Work out the finished part from the listing and answer in its coordinate system (mm). A direction names the side the tool comes from. Round coordinates to 2 decimals unless told otherwise and drop trailing zeros. Write each loop counter-clockwise with the first axis right and the second up, starting at its lowest first coordinate (ties: lowest second). Pieces come first, ordered by that corner, then holes.
from build123d import *

# Parameters (mm, degrees)
SKETCH_263_W        = 2284
SKETCH_263_H        = 90
EXTRUDE_4_DEPTH     = 8
SKETCH_3_W          = 2284
SKETCH_3_H          = 9
EXTRUDE_5_DEPTH     = 72
SKETCH_4_R          = 11
CUT_EXTRUDE_2_DEPTH = 2287.835586569


with BuildPart() as part:
    # Sketch 263 → 拉伸4 (new body)
    with BuildSketch(Plane.XY):
        with Locations((1142, 45)):
            Rectangle(SKETCH_263_W, SKETCH_263_H)
    extrude(amount=EXTRUDE_4_DEPTH)

    # 草图3 → 拉伸5 (add)
    with BuildSketch(Plane.XY.offset(8)):
        with Locations((1142, 4.5)):
            Rectangle(SKETCH_3_W, SKETCH_3_H)
    extrude(amount=EXTRUDE_5_DEPTH)

    # 草图4 → 切除-拉伸2 (cut, through all)
    with BuildSketch(Plane(origin=(0, 9, 0), x_dir=(1, 0, 0), z_dir=(0, 1, 0))):
        with Locations(Location((39.95, -40, 0), (0, 0, 270))):
            Circle(SKETCH_4_R)
        with Locations(Location((109.95, -40, 0), (0, 0, 270))):
            Circle(SKETCH_4_R)
        with Locations(Location((2174.05, -40, 0), (0, 0, 270))):
            Circle(SKETCH_4_R)
        with Locations(Location((2244.05, -40, 0), (0, 0, 270))):
            Circle(SKETCH_4_R)
    extrude(amount=-CUT_EXTRUDE_2_DEPTH, mode=Mode.SUBTRACT)


solid = part.part
Q1. Find the intervals of material crossed by L1, parallel to X at y = 2, z = 40; L2, parallel to Z at x = 2174, y = 6; L3, parallel to Y at x = 2150, z = 37, in increasing order.
Q2. Find section B-B (y = 46.5). Determine the outline of the cut face in (x, z).
Q3. Given pin 1 (20 mm diameter, centred on x = 39.95, z = 40, fed in from -Y), flat-ended and moving along its own axis, determine where the tip first touches the part or whether it passes through.
Q4. A tool of negligible diameter and unlimited length cuts with its end or side. For faces 1 (the face through (1126, 50, 8)), 2 (the face through (2284, 25, 7)), from which of +Z, -Z, +X, -X, +Y, -Y can it reach the whole face along a straight path? Write none if from no direction.
Q5. Find section A-A (x = 1153). Determine the outline of the cut face in (y, z), plus the area to 3 significant figures.
Report:
1. L1: x = 0 to 28.95, 50.95 to 98.95, 120.95 to 2163.05, 2185.05 to 2233.05, 2255.05 to 2284
1. L2: z = 0 to 29, 51 to 80
1. L3: y = 0 to 9
2. outline: (0, 0) - (2284, 0) - (2284, 8) - (0, 8) - close
3. pin 1: passes through
4. face 1: +Z, +X, -X, +Y
4. face 2: +Z, -Z, +X, +Y, -Y
5. outline: (0, 0) - (90, 0) - (90, 8) - (9, 8) - (9, 80) - (0, 80) - close
5. area: 1,370 mm2
